Source: CAD feature listing. Evaluate the final solid. Frame: model axes, mm. Face numbers are marked on the shaded views. Give positions to 0.01 mm unless a question says otherwise; leave off trailing zeros. Loops run counter-clockwise (first coordinate to the right, second up) from the corner with the lowest first, then second, coordinate; pieces in that order, holes last. Notation, with made-up numbers: M 14.25,24.5 L 32.25,24.5 A17 cw 32.25,44.5 Z; hole C -18.5,66.25 d3. An arc over 180 degrees is marked long. Answer in a Markdown table with one row per item.
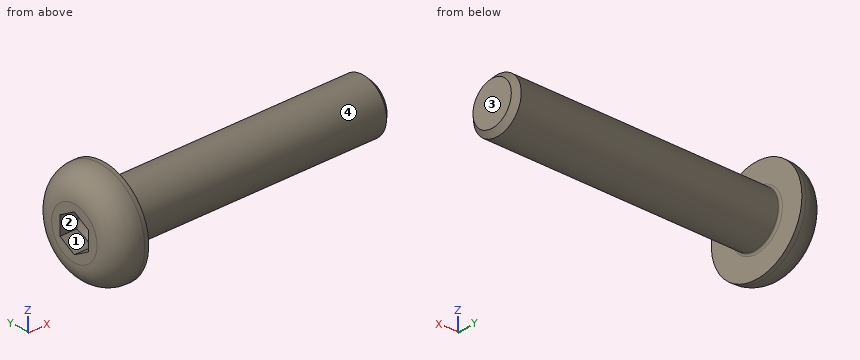
Autodesk Inventor part; units mm, degrees
ref_plane "Work Plane1" through (30, 0, 0) normal (0, -0.5, 0.866) x (1, 0, 0)
ref_plane "YZ Plane" through (0, 0, 0) normal (1, 0, 0) x (0, 1, 0)
ref_plane "XZ Plane" through (0, 0, 0) normal (0, 1, 0) x (-1, 0, 0)
sketch "Sketch1" plane through (0, 0, 0) normal (0, 0, 1) x (1, 0, 0)
  line L0 (-0.19, 0) -> (25, 0)
  line L1 (25, 0) -> (25, 2.5)
  line L2 (25, 2.5) -> (1.6, 2.5)
  line L3 (1.6, 2.5) -> (1.1092, 2.5)
  line L4 (1.1092, 2.5) -> (0, 2.5)
  line L5 (0, 2.5) -> (0, 4.75)
  line L6 (0, 4.75) -> (-2.75, 4.75)
  line L7 (-2.75, 4.75) -> (-2.75, 1.7321)
  line L8 (-2.75, 1.7321) -> (-1.19, 1.7321)
  line L9 (-1.19, 1.7321) -> (-0.19, 0)
  line L10 (-8.3, 0) -> (30.55, 0)
  line L11 (0, -0.95) -> (0, 5.7)
  line L12 (1.6, 2.5) -> (0, 2.5) construction
  dimension "d0" = 23.4
  dimension "d1" = 0.4908
  dimension "d2" = 2.75
  dimension "d3" = 1.56
  dimension "d4" = 60
  dimension "d5" = 5
  dimension "d6" = 5
  dimension "d7" = 3.4641
  dimension "d8" = 9.5
  dimension "d19" = 25
revolve "Body" add sketch "Sketch1" angle 360 about axis through (-0.19, 0, 0) along (1, 0, 0)
sketch "Sketch2" plane through (-2.75, 0, 0) normal (-1, 0, 0) x (0, 0, 1)
  circle A0 centre (0, 0) radius 1.7321
  line L0 (0, -6.65) -> (0, 6.65)
  line L1 (-6.65, 0) -> (6.65, 0)
  line L2 (1.7321, 0) -> (0.866, -1.5)
  line L3 (0.866, -1.5) -> (-0.866, -1.5)
  line L4 (-0.866, -1.5) -> (-1.7321, 0)
  line L5 (-1.7321, 0) -> (-0.866, 1.5)
  line L6 (-0.866, 1.5) -> (0.866, 1.5)
  line L7 (0.866, 1.5) -> (1.7321, 0)
extrude "Slot" add sketch "Sketch2" against normal up to next contours L7 A0 | A0 L2 | L6 L0 A0 | A0 L0 L3 | L0 L6 A0 | A0 L3 L0 | L4 A0 | A0 L5
fillet "Fillet1" radius 2.375 1 edges at (-2.75, -4.75, 0)
thread "Thread"
chamfer "Chamfer1" distance 0.4908 distance2 0.4908 1 edges at (25, -2.5, 0) measured on face at (25, -0.5525, -0.0341)
fillet "Fillet2" radius 0.2 1 edges at (0, -2.5, 0)
ref_plane "Work Plane1" through (30, 0, 0) normal (0, -0.5, 0.866) x (1, 0, 0)
equation "\"d0\" = GEL"
equation "\"d1\" = GAL"
equation "\"d2\" = KOH"
equation "\"d3\" = INTI"
equation "\"d5\" = GD"
equation "\"d6\" = BDM"
equation "\"d7\" = 1.1547 * SW"
equation "\"d8\" = KOD"
equation "\"d19\" = NLG"
equation "\"d16\" = RR"
equation "\"d12\" = GEL"
equation "\"d14\" = -0.5 * SPD + 0.5 * GD"
equation "\"d15\" = GUL"
equation "\"d29\" = R"
equation "\"GD\" = NND"
equation "\"NLG\" = 25"
equation "\"GEL\" = 23.4"
equation "\"KOD\" = 9.5"
equation "\"KOH\" = 2.75"
equation "\"INTI\" = 1.56"
equation "\"GAL\" = 0.61345 * PTC"
equation "\"GUL\" = 0.61345 * PTC"
equation "\"BDM\" = NND"
equation "\"SW\" = 3"
equation "\"RR\" = 2.375"
equation "\"SPD\" = 4.01848"
equation "\"d28\" = R"
equation "\"R\" = 0.2"
equation "\"TOA\" = 30deg"
equation "\"THREADDIA\" = 5"
equation "\"KOD1\" = KOD - 2 * RR"
equation "\"PTC\" = 0.8"
equation "\"NND\" = 5"
equation "\"E0\" = 1.155 * SW"
equation "\"GD1\" = THREADDIA - 1.2269 * PTC"
properties part number "ANSI B18.3.4M - M5 x 0.8 x 25"
1) Pull-direction query (Z, two-part tool) for the marked faces 1, 2, 3 and 4; classes: released by +Z, released by -Z, zero draft, split by the parting line, or undercut.
Reply:
| item | result |
|---|---|
| face 1 | undercut |
| face 2 | undercut |
| face 3 | zero draft |
| face 4 | split by the parting line |
2) Pin query (flat end, axial travel): pin 1 Ø0.5 at (x, z) = (-1.5, 0) entering from -Y; pin 2 Ø1.5 at (x, z) = (5, -1.5) entering from -Y; pin 3 Ø1.5 at (x, y) = (3.5, -0.5) entering from -Z. Return the tip coordinate at first contact, or that it passes through.
Reply:
| item | result |
|---|---|
| pin 1 | stops at y = -4.58 |
| pin 2 | stops at y = -2.38 |
| pin 3 | stops at z = -2.5 |
3) Material intervals for L1, parallel to Z at x = 11, y = 0; L2, parallel to Y at x = 14.25, z = -1.5; L3, parallel to Y at x = 4, z = 0.5, sorted ascending.
Reply:
| item | result |
|---|---|
| L1 | z = -2.5 to 2.5 |
| L2 | y = -2 to 2 |
| L3 | y = -2.45 to 2.45 |
4) Section A-A, the plane x = 22. Return loops of the section in (y, z).
Reply:
| item | result |
|---|---|
| outline | C 0,0 d5 |
